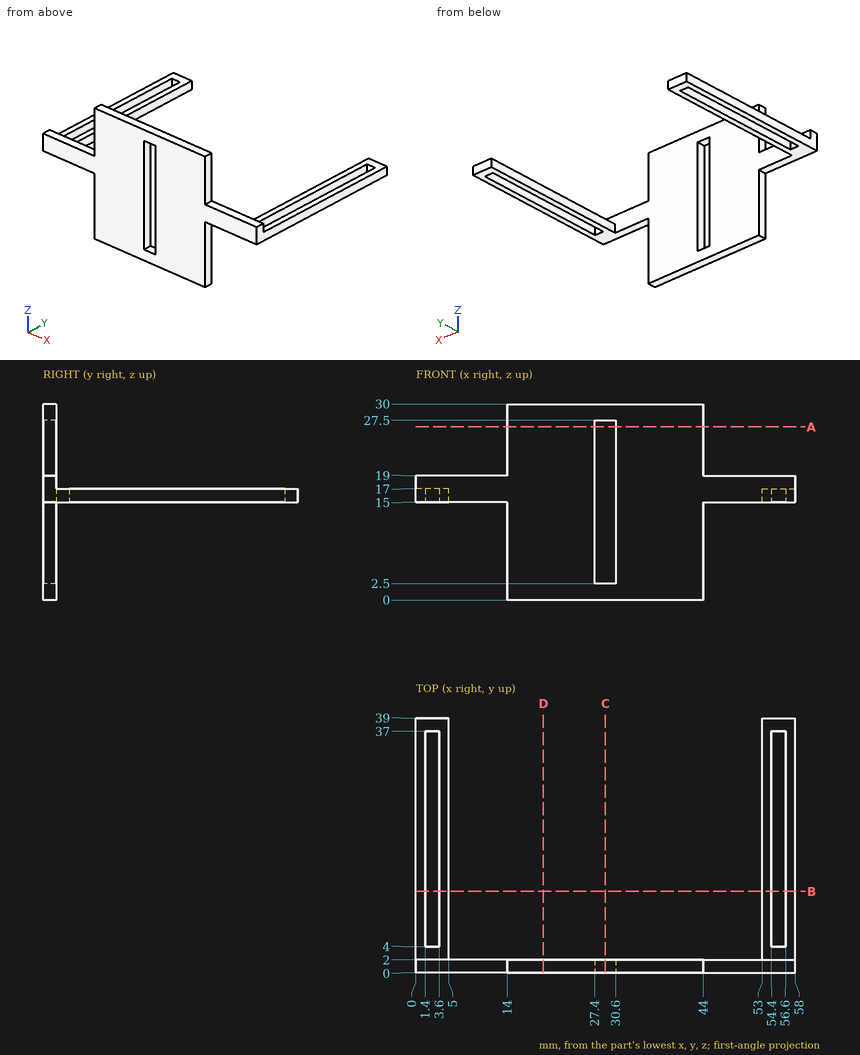
Verification items for this drawing (mm, ordinates from the low corner). Give positions to 0.01 mm unless a question says otherwise; leave off trailing zeros. Loops run counter-clockwise (first coordinate to the right, second up) from the corner with the lowest first, then second, coordinate; pieces in that order, holes last. Notation, with made-up numbers: M 2,15.5 L 37,15.5 A17 cw 37,30.5 Z; hole C 28,15.5 d11. An arc over 180 degrees is marked long. Write item = value, one per line.
(1) Gauge pin test, flat ends, axial feed: pin 1 Ø4 at (x, z) = (47.5, 8) entering from -Y; pin 2 Ø15 at (x, z) = (43.5, 9.5) entering from +Y; pin 3 Ø12 at (y, z) = (23.5, 13.5) entering from +X; pin 4 Ø0.6 at (x, y) = (51.5, 0.5) entering from +Z. Record the tip position at first contact, or that the pin passes through.
Answer below:
pin_1 = through
pin_2 = 2
pin_3 = 58
pin_4 = 19
(2) Sectioned sample at D-D, the plane x = 19.5. Record the cut outline in (y, z).
Answer below:
outline = M 0,0 L 2,0 L 2,30 L 0,30 Z
(3) Sectioned sample at A-A, the plane z = 26.5. Record the cut outline in (x, y).
Answer below:
outline = M 14,0 L 27.4,0 L 27.4,2 L 14,2 Z; M 30.6,0 L 44,0 L 44,2 L 30.6,2 Z
(4) Sectioned sample at C-C, the plane x = 29. Record the cut outline in (y, z), plus the area to 3 significant figures.
Answer below:
outline = M 0,0 L 2,0 L 2,2.5 L 0,2.5 Z; M 0,27.5 L 2,27.5 L 2,30 L 0,30 Z
area = 10.0 mm2
(5) Sectioned sample at B-B, the plane y = 12.5. Record the cut outline in (x, z), plus the area to 3 significant figures.
Answer below:
outline = M 0,15 L 1.4,15 L 1.4,17 L 0,17 Z; M 3.6,15 L 5,15 L 5,17 L 3.6,17 Z; M 53,15 L 54.4,15 L 54.4,17 L 53,17 Z; M 56.6,15 L 58,15 L 58,17 L 56.6,17 Z
area = 11.2 mm2
(6) Material ranges on line 1 (X direction, y = 6.5, z = 15.5); line 2 (Y direction, x = 8, z = 17.5), recorded low to high. Write a range as [from, to].
Answer below:
line_1 = [0, 1.4], [3.6, 5], [53, 54.4], [56.6, 58]
line_2 = [0, 2]
